Geometry check sheet. Reference: the model listing, model coordinates, mm. A direction names the side the tool comes from. Coordinates: 2 decimals unless noted, no trailing zeros. Loops run counter-clockwise (first coordinate to the right, second up) from the corner with the lowest first, then second, coordinate; pieces in that order, holes last. Notation, with made-up numbers: (84.5, -12) - (122.5, -12) arc R9 ccw to (122.5, 5) - close; hole circle Ø6 at (52, 77). An arc over 180 degrees is marked (long way). One line per item, written item: value.
from build123d import *

# Parameters (mm, degrees)
SKETCH1_R               = 21
BOSS_EXTRUDE1_DEPTH     = 42
BOSS_EXTRUDE2_DEPTH     = 12
BOSS_EXTRUDE5_DEPTH     = 70
SKETCH2_W               = 35
SKETCH2_H               = 22
CUT_EXTRUDE2_DEPTH      = 70
CUT_EXTRUDE4_DEPTH      = 1
CUT_EXTRUDE4_DEPTH_BACK = 25
SKETCH5_W               = 6
SKETCH5_H               = 18
BOSS_EXTRUDE6_DEPTH     = 33
FILLET1_R               = 5
SKETCH8_W               = 25
SKETCH8_H               = 6
CUT_EXTRUDE6_DEPTH      = 167
SKETCH7_R               = 7.5
CUT_EXTRUDE7_DEPTH      = 167
SKETCH7_3_R             = 12.5
CUT_EXTRUDE8_DEPTH      = 7
FILLET2_R               = 20
SKETCH7_4_R             = 12.5
SKETCH7_4_R_2           = 7.5
CUT_EXTRUDE9_DEPTH      = 7
SKETCH7_5_R             = 7.5
CUT_EXTRUDE10_DEPTH     = 21
SKETCH11_R              = 5
CUT_EXTRUDE11_DEPTH     = 80


with BuildPart() as part:
    # Sketch1 → Boss-Extrude1 (new body)
    with BuildSketch(Plane.XY):
        Circle(SKETCH1_R)
    extrude(amount=BOSS_EXTRUDE1_DEPTH)

    # Sketch1<3> → Boss-Extrude2 (add)
    with BuildSketch(Plane.XY):
        with BuildLine():
            ThreePointArc((21, 0), (-6.343349758, -20.019038784), (-17.167801318, 12.094072841))
            Line((-17.167801318, 12.094072841), (-75, -70))
            Line((-75, -70), (52.5, -70))
            Line((52.5, -70), (52.5, -52))
            ThreePointArc((52.5, -52), (70, -34.5), (87.5, -52))
            Line((87.5, -52), (87.5, -70))
            Line((87.5, -70), (99, -70))
            Line((99, -70), (99, -30))
            Line((99, -30), (10.043243118, 18.442702288))
            ThreePointArc((10.043243118, 18.442702288), (18.054197649, 10.725947383), (21, 0))
        make_face()
    extrude(amount=BOSS_EXTRUDE2_DEPTH)

    # Sketch1<7> → Boss-Extrude5 (add)
    with BuildSketch(Plane.XY):
        with BuildLine():
            Line((52.5, -70), (-75, -70))
            Line((-75, -70), (-75, -90))
            Line((-75, -90), (105, -90))
            Line((105, -90), (105, -30))
            Line((105, -30), (99, -30))
            Line((99, -30), (99, -70))
            Line((99, -70), (87.5, -70))
            Line((87.5, -70), (87.5, -52))
            ThreePointArc((87.5, -52), (70, -34.5), (52.5, -52))
            Line((52.5, -52), (52.5, -70))
        make_face()
    extrude(amount=BOSS_EXTRUDE5_DEPTH)

    # Sketch2 → Cut-Extrude2 (cut)
    with BuildSketch(Plane(origin=(0, 0, 0), x_dir=(1, 0, 0), z_dir=(0, 1, 0))):
        with Locations((70, -23)):
            Rectangle(SKETCH2_W, SKETCH2_H)
    extrude(amount=-CUT_EXTRUDE2_DEPTH, mode=Mode.SUBTRACT)

    # Sketch3 → Cut-Extrude4 (cut, two sides)
    with BuildSketch(Plane.XY.offset(70)) as cut_extrude4_sk:
        with BuildLine():
            Line((57.5, -52), (57.5, -90))
            Line((57.5, -90), (82.5, -90))
            Line((82.5, -90), (82.5, -52))
            ThreePointArc((82.5, -52), (70, -39.5), (57.5, -52))
        make_face()
    extrude(amount=CUT_EXTRUDE4_DEPTH, mode=Mode.SUBTRACT)
    extrude(cut_extrude4_sk.sketch, amount=-CUT_EXTRUDE4_DEPTH_BACK, mode=Mode.SUBTRACT)

    # Sketch5 → Boss-Extrude6 (add)
    with BuildSketch(Plane.XY.offset(45)):
        with Locations((70, -61)):
            Rectangle(SKETCH5_W, SKETCH5_H)
    extrude(amount=-BOSS_EXTRUDE6_DEPTH)

    # Fillet1
    fillet1_edges = [part.edges().sort_by_distance(p)[0] for p in [
        (102, -30, 70),
    ]]
    fillet(fillet1_edges, radius=FILLET1_R)

    # Sketch8 → Cut-Extrude6 (cut)
    with BuildSketch(Plane.XY.offset(45)):
        with Locations((70, -87)):
            Rectangle(SKETCH8_W, SKETCH8_H)
    extrude(amount=-CUT_EXTRUDE6_DEPTH, mode=Mode.SUBTRACT)

    # Sketch7 → Cut-Extrude7 (cut)
    with BuildSketch(Plane(origin=(0, -70, 0), x_dir=(1, 0, 0), z_dir=(0, 1, 0))):
        with Locations((-55, -50)):
            Circle(SKETCH7_R)
    extrude(amount=-CUT_EXTRUDE7_DEPTH, mode=Mode.SUBTRACT)

    # Sketch7<3> → Cut-Extrude8 (cut)
    with BuildSketch(Plane(origin=(0, -70, 0), x_dir=(1, 0, 0), z_dir=(0, 1, 0))):
        with Locations((-55, -50)):
            Circle(SKETCH7_3_R)
    extrude(amount=-CUT_EXTRUDE8_DEPTH, mode=Mode.SUBTRACT)

    # Fillet2
    fillet2_edges = [part.edges().sort_by_distance(p)[0] for p in [
        (-75, -80, 70),
    ]]
    fillet(fillet2_edges, radius=FILLET2_R)

    # Sketch7<4> → Cut-Extrude9 (cut)
    with BuildSketch(Plane(origin=(0, -70, 0), x_dir=(1, 0, 0), z_dir=(0, 1, 0))):
        with Locations((5, -50)):
            Circle(SKETCH7_4_R)
        with Locations((5, -50)):
            Circle(SKETCH7_4_R_2, mode=Mode.SUBTRACT)
    extrude(amount=-CUT_EXTRUDE9_DEPTH, mode=Mode.SUBTRACT)

    # Sketch7<5> → Cut-Extrude10 (cut, through all)
    with BuildSketch(Plane(origin=(0, -70, 0), x_dir=(1, 0, 0), z_dir=(0, 1, 0))):
        with Locations((5, -50)):
            Circle(SKETCH7_5_R)
    extrude(amount=-CUT_EXTRUDE10_DEPTH, mode=Mode.SUBTRACT)

    # Sketch10 → Cut-Revolve1 (revolve, cut)
    with BuildSketch(Plane(origin=(0, 0, 0), x_dir=(1, 0, 0), z_dir=(0, 1, 0))):
        Polygon((0, 0), (0, -42.225297228), (13.5, -42.225297228), (13.5, -20.830460942), (7.5, -17.225297228), (7.5, 0), align=None)
    revolve(axis=Axis((0, 0, 0), (0, 0, 1)), mode=Mode.SUBTRACT)

    # Sketch11 → Cut-Extrude11 (cut)
    with BuildSketch(Plane(origin=(0, 0, 0), x_dir=(1, 0, 0), z_dir=(0, 1, 0))):
        with Locations((70, -55)):
            Circle(SKETCH11_R)
    extrude(amount=-CUT_EXTRUDE11_DEPTH, mode=Mode.SUBTRACT)


solid = part.part
(1) Cross-section at D-D on y = -44. Record the cut outline in (x, z), and give its area (3 significant figures).
Reply:
outline: (-56.68, 0) - (105, 0) - (105, 70) - (99, 70) - (99, 12) - (-56.68, 12) - close; (54.44, 34) - (85.56, 34) - (85.56, 70) - (79.6, 70) - (79.6, 45) - (60.4, 45) - (60.4, 70) - (54.44, 70) - close
area: 2,930 mm2
(2) Release check for a two-part mould opening along Y. For faces 1 (the face through (2.29, -73.451, 62.203)), 2 (the face through (-47, -77, 50)), 3 (the face through (73, -61, 23)), 4 (the face through (70, -84, 23)) record: pulls with the +Y half, pulls with the -Y half, needs draft (parallel to the pull), parting line crosses it, or undercut.
Reply:
face 1: undercut
face 2: pulls with the +Y half
face 3: needs draft
face 4: pulls with the -Y half
(3) Cross-section at B-B on x = 70. Record the cut outline in (y, z).
Reply:
outline: (-84, 0) - (-14.21, 0) - (-14.21, 12) - (-52, 12) - (-52, 34) - (-34.5, 34) - (-34.5, 50) - (-39.5, 50) - (-39.5, 45) - (-84, 45) - close; (-39.5, 60) - (-34.5, 60) - (-34.5, 70) - (-39.5, 70) - close
(4) Access from +Z, -Z, +X, -X, +Y, -Y to the whole of each face (thin tool, end or side, straight path). Record for faces 5 (the face through (-67.488, -73.451, 49.45)), 6 (the face through (5, -77, 58)), 7 (the face through (70.385, -34.504, 47.748)), 8 (the face through (67, -61, 23)), 9 (the face through (82.5, -75, 51)).
Reply:
face 5: +Y
face 6: none
face 7: +Z, +Y
face 8: -X, +Y
face 9: +Z, -Y
(5) Cross-section at A-A on z = 9. Record the cut outline in (x, y), and give its area (3 significant figures).
Reply:
outline: (-75, -90) - (57.5, -90) - (57.5, -84) - (82.5, -84) - (82.5, -90) - (105, -90) - (105, -30) - (99, -30) - (10.04, 18.44) arc R21 ccw to (-17.17, 12.09) - (-75, -70) - close; hole circle Ø15 at (0, 0)
area: 14,000 mm2
(6) Go/stop test with flat-tipped pins: pin 1 Ø8 at (y, z) = (-65.5, 19) entering from -X; pin 2 Ø3 at (x, z) = (46.5, 16) entering from +Y; pin 3 Ø12.5 at (x, z) = (66.5, 13.5) entering from -Y. Record where each tip stops, or that it passes through.
Reply:
pin 1: x = 67
pin 2: y = -70
pin 3: y = -84
(7) Material ranges on probe 1 along X at (y, z) = (-74, 50); probe 2 along Z at (x, y) = (-55, -85); probe 3 along X at (y, z) = (-62.5, 46.5), recorded low to high. Write a range as from..to.
Reply:
probe 1: -75..-67.5, -42.5..-7.5, 17.5..57.5, 82.5..105
probe 2: 0..42.5, 57.5..70
probe 3: 52.5..57.5, 82.5..87.5, 99..105
(8) Cross-section at C-C on x = 0. Record the cut outline in (y, z).
Reply:
outline: (-90, 0) - (-7.5, 0) - (-7.5, 17.23) - (-13.5, 20.83) - (-13.5, 42) - (-21, 42) - (-21, 12) - (-70, 12) - (-70, 38.54) - (-77, 38.54) - (-77, 44.41) - (-90, 44.41) - close; (-90, 55.59) - (-77, 55.59) - (-77, 61.46) - (-70, 61.46) - (-70, 70) - (-90, 70) - close; (7.5, 0) - (21, 0) - (21, 42) - (13.5, 42) - (13.5, 20.83) - (7.5, 17.23) - close
